Geometry check sheet. Reference: the model listing, model coordinates, mm. Face numbers are marked on the shaded views. A direction names the side the tool comes from. Coordinates: 2 decimals unless noted, no trailing zeros. Write each loop counter-clockwise with the first axis right and the second up, starting at its lowest first coordinate (ties: lowest second). Pieces come first, ordered by that corner, then holes. Notation, with made-up numbers: M -36,43.25 L 20,43.25 A11 ccw 20,54.25 Z; hole C 17.25,72.25 d5. An arc over 180 degrees is marked long. Put each result on its own line as item: value. Start each with the question number.
1) Cross-section at B-B on z = -19.5. Record the cut outline in (x, y).
2) Set-up check for the marked faces 1, 2 and 3: record each of +Z, -Z, +X, -X, +Y, -Y from which the full face is reachable in a straight line by a thin tool's end or side.
3) Cross-section at D-D on z = -5. Record the cut outline in (x, y), plus the area to 3 significant figures.
4) Cross-section at A-A on x = 0. Record the cut outline in (y, z), plus the area to 3 significant figures.
5) Mould release check, pull along Y, two halves, no side actions. Record for the marked faces 4 and 5: released by +Y, released by -Y, zero draft, split by the parting line, or undercut.
6) Scan lines: line 1 along X through (y, z) = (0, -11.2); line 2 along X through (y, z) = (0, -33.5); line 3 along Y through (x, z) = (-3, -59). Record each from-to range of solid material in increasing order.
7) Cross-section at C-C on x = -21. Record the cut outline in (y, z), plus the area to 3 significant figures.
8) Gauge pin test, flat ends, axial feed: pin 1 (10 mm diameter, centred on x = 26, z = -29.5, fed in from +Y); pin 2 (4 mm diameter, centred on y = 11, z = -22.5, fed in from -X); pin 3 (3 mm diameter, centred on y = -5, z = -21, fed in from +X); pin 4 (4 mm diameter, centred on x = -6, z = -57.5, fed in from +Y). Record the tip position at first contact, or that the pin passes through.
Autodesk Inventor part; units mm, degrees
ref_plane "Plan de construction1" through (16.5, 0, -15) normal (1, 0, 0) x (0, 1, 0)
ref_plane "XZ Plane" through (0, 0, 0) normal (0, 1, 0) x (-1, 0, 0)
ref_plane "XY Plane" through (0, 0, 0) normal (0, 0, 1) x (1, 0, 0)
sketch "Esquisse1" plane through (0, 0, 0) normal (1, 0, 0) x (0, 1, 0)
  line L0 (0, 0) -> (0, -16.8642)
  line L1 (12.75, -0.5) -> (12.75, -10) construction
  line L2 (13, -0.5) -> (13, -10)
  line L3 (13.5, 0) -> (16.25, 0)
  line L4 (16.25, 0) -> (16.5, -0.25)
  line L5 (16.5, -0.25) -> (16.5, -29.75)
  line L6 (12.75, -64.25) -> (12.75, -12)
  line L7 (13, -10) -> (11.25, -10)
  line L8 (12.75, -12) -> (11.25, -12)
  line L9 (11.25, -10) -> (11.25, -12)
  line L10 (11, -10) -> (11, -12) construction
  line L11 (13.5, 0) -> (13, -0.5)
  line L12 (12.5, -12) -> (12.5, -64.25) construction
  line L13 (12.5, -0.5) -> (12.5, -10) construction
  line L14 (16.5, -29.75) -> (17.25, -39.75)
  line L15 (17.25, -39.75) -> (17.75, -40.25)
  line L16 (17.75, -40.25) -> (18.75, -40.25)
  line L17 (18.75, -40.25) -> (18.75, -44.25)
  line L18 (18.75, -44.25) -> (12.75, -64.25)
  dimension "d2" = 0.25
  dimension "d3" = 0.25
  dimension "d8" = 33
  dimension "d9" = 0.25
  dimension "d13" = 0.25
  dimension "d14" = 22
  dimension "d15" = 10
  dimension "d16" = 0.5
  dimension "d17" = 0.5
  dimension "d18" = 25
  dimension "d19" = 0.25
  dimension "d20" = 2
  dimension "d21" = 0.25
  dimension "d22" = 25
  dimension "d23" = 0.5
  dimension "d24" = 10
  dimension "d25" = 0.75
  dimension "d26" = 0.5
  dimension "d28" = 40.25
  dimension "d45" = 64.25
  dimension "d51" = 1
  dimension "d52" = 20
  dimension "d54" = 4
revolve "Révolution1" add sketch "Esquisse1" angle 360 about axis through (0, 0, 0) along (0, 0, -1)
ref_plane "Plan de construction1" through (16.5, 0, -15) normal (1, 0, 0) x (0, 1, 0)
sketch "Esquisse2" plane through (16.5, 0, -15) normal (1, 0, 0) x (0, 1, 0)
  circle A0 centre (0, 1.5) radius 3
  line L0 (0, -62.1) -> (0, 27.85)
  line L1 (-16.25, 15) -> (16.25, 15)
  point P0 (0, 15)
  dimension "d29" = 6
  dimension "d30" = 13.5
extrude "Extrusion1" add sketch "Esquisse2" along normal blind 20 and the other way blind 0.5
chamfer "Chanfrein1" distance 0.5 angle 45 4 edges at (36.5, -3, -13.5) (16.3413, 2.2832, -11.554) (16.225, -3, -13.4926) (16.3418, 2.2797, -15.4502)
pattern_circular "Réseau circulaire1" count 2 over 360 about axis through (0, 0, -10) along (0, 0, 1) of "Extrusion1", "Chanfrein1"
equation "\"d3\" = d2"
equation "\"d17\" = d16"
properties part number "canon_support_entree"
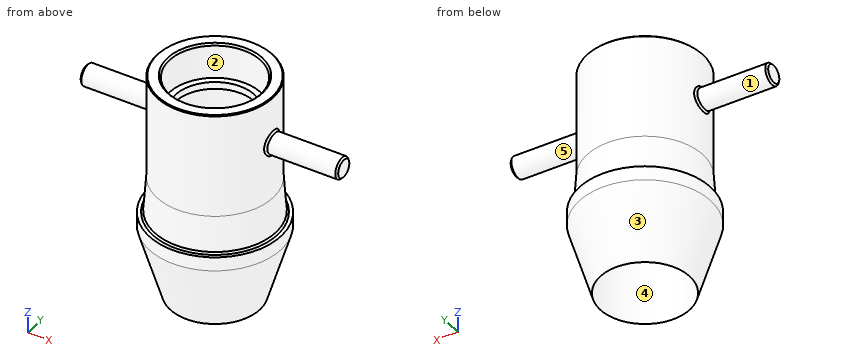
Answer key:
1. outline: C 0,0 d33; hole C 0,0 d25.5
2. face 1: -X
2. face 2: +Z
2. face 3: -Z
3. outline: C 0,0 d33; hole C 0,0 d26
3. area: 324 mm²
4. outline: M -18.75,-44.25 L -12.75,-64.25 L -12.75,-12 L -11.25,-12 L -11.25,-10 L -13,-10 L -13,-0.5 L -13.5,0 L -16.25,0 L -16.5,-0.25 L -16.5,-29.75 L -17.25,-39.75 L -17.75,-40.25 L -18.75,-40.25 Z; M 11.25,-12 L 12.75,-12 L 12.75,-64.25 L 18.75,-44.25 L 18.75,-40.25 L 17.75,-40.25 L 17.25,-39.75 L 16.5,-29.75 L 16.5,-0.25 L 16.25,0 L 13.5,0 L 13,-0.5 L 13,-10 L 11.25,-10 Z
4. area: 479 mm²
5. face 4: undercut
5. face 5: split by the parting line
6. line 1: x = -36.5 to -11.25, 11.25 to 36.5
6. line 2: x = -16.78 to -12.75, 12.75 to 16.78
6. line 3: y = -14.01 to -12.39, 12.39 to 14.01
7. outline: C 0,-13.5 d6
7. area: 28.3 mm²
8. pin 1: passes through
8. pin 2: stops at x = -13.83
8. pin 3: stops at x = 16.12
8. pin 4: stops at y = 14.49
